Study the drawing (mm; zero at the part's minimum x, y, z) and answer. Give positions to 0.01 mm unless a question says otherwise; leave off trailing zeros. Loops run counter-clockwise (first coordinate to the right, second up) from the corner with the lowest first, then second, coordinate; pieces in that order, holes last. Notation, with made-up numbers: M 12,-34 L 39,-34 A31 cw 39,-9 Z; hole C -37,-18.5 d11. An arc over 180 degrees is marked long. Return JSON: item names as keys, results as strings.
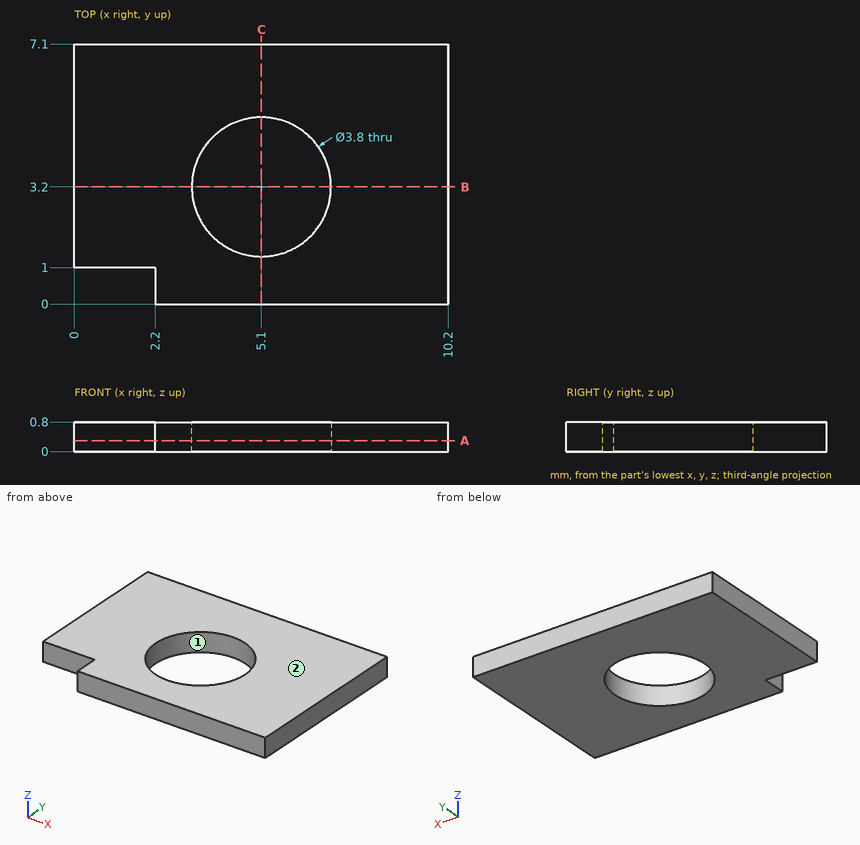
(1) The part is cut by section C-C (x = 5.1). Determine the outline of the cut face in (y, z), and give its area (3 significant figures).
Values follow:
{"outline": "M 0,0 L 1.3,0 L 1.3,0.8 L 0,0.8 Z; M 5.1,0 L 7.1,0 L 7.1,0.8 L 5.1,0.8 Z", "area": "2.64 mm²"}
(2) Determine the mould class of the marked faces 1 and 2 for opening direction Y: released by +Y, released by -Y, zero draft, split by the parting line, or undercut.
Values follow:
{"face 1": "undercut", "face 2": "zero draft"}
(3) The part is cut by section B-B (y = 3.2). Determine the outline of the cut face in (x, z), and give its area (3 significant figures).
Values follow:
{"outline": "M 0,0 L 3.2,0 L 3.2,0.8 L 0,0.8 Z; M 7,0 L 10.2,0 L 10.2,0.8 L 7,0.8 Z", "area": "5.12 mm²"}
(4) Straight lines are drawn through the part: line 1 along Y through (x, z) = (5.1, 0.3); line 2 along X through (y, z) = (2.25, 0.55); line 3 along X through (y, z) = (2, 0.75). For each, find the intervals that lie inside material, in ascending order.
Values follow:
{"line 1": "0 to 1.3, 5.1 to 7.1", "line 2": "0 to 3.45, 6.75 to 10.2", "line 3": "0 to 3.63, 6.57 to 10.2"}
(5) The part is cut by section A-A (z = 0.3). Determine the outline of the cut face in (x, y), and give its area (3 significant figures).
Values follow:
{"outline": "M 0,1 L 2.2,1 L 2.2,0 L 10.2,0 L 10.2,7.1 L 0,7.1 Z; hole C 5.1,3.2 d3.8", "area": "58.9 mm²"}
